```python
from build123d import *

# Parameters (mm, degrees)
F0_W     = 250
F0_H     = 100
F1_DEPTH = 5
F4_DEPTH = 50
F5_R     = 5
F6_R     = 4.99999


# Not quite as in the source:
# - two fillets or chamfers of one size are made in one step
# - a fillet or chamfer is up to 0.001 mm smaller than in the source, because OpenCascade refuses the exact size


with BuildPart() as f1:
    # F0 (on Front) → F1 (new body, symmetric)
    with BuildSketch(Plane.XZ):
        Rectangle(F0_W, F0_H)
    extrude(amount=F1_DEPTH, both=True)

    # F3 (on Top) → F4 (join, symmetric)
    with BuildSketch(Plane.XY):
        Polygon((-55.8243768029, -21.1299679096), (-77.5685643683, -5), (-94.3532884121, -5), (-61.7821750806, -29.1614459605), align=None)
    extrude(amount=F4_DEPTH, both=True)

    # F5
    f5_edges = [f1.edges().sort_by_distance(p)[0] for p in [
        (-94.353288, -5, 0),
        (-77.568564, -5, 0),
    ]]
    fillet(f5_edges, radius=F5_R)

    # F6 (radius 5 in the source; OpenCascade refuses exactly that, so slightly less here)
    f6_edges = [f1.edges().sort_by_distance(p)[0] for p in [
        (-61.782175, -29.161446, 0),
        (-55.824377, -21.129968, 0),
    ]]
    fillet(f6_edges, radius=F6_R)


solid = f1.part
```
Source: CAD feature listing. Evaluate the final solid. Frame: model axes, mm. A direction names the side the tool comes from. Round coordinates to 2 decimals unless told otherwise and drop trailing zeros. Loops run counter-clockwise (first coordinate to the right, second up) from the corner with the lowest first, then second, coordinate; pieces in that order, holes last. Notation, with made-up numbers: M -30,33.5 L -6,33.5 A28 ccw -6,56.5 Z; hole C -15.5,40 d6. An arc over 180 degrees is marked long. Use a Markdown table: item, result. Add a question column.
1. Section query B-B on x = -10. Return the cut outline in (y, z).
2. Line query: line 1 (Y direction, x = 87.5, z = -14); line 2 (Y direction, x = -63, z = 13); line 3 (X direction, y = -12.5, z = -29). Output: solid intervals per line, ascending.
3. Mould query, pull axis Y, two halves, no side actions, for faces 1 (the cylindrical face through (-62, -27.1, -0.7)), 2 (the cylindrical face through (-67.155, -8.348, 0.7)), 3 (the flat face through (-10, -2, 50)), 4 (the flat face through (-62.59, -16.11, 0.7)). Classes: pulls with the +Y half, pulls with the -Y half, needs draft (parallel to the pull), parting line crosses it, or undercut.
4. Contact query for flat-ended pins moving along their axis: P1, Ø10, axis at x = -66, z = -6, coming from the -Y side; P2, Ø14.5, axis at x = -104, z = -6.5, coming from the -Y side. Output: stop coordinate, or through.
5. Section query C-C on y = -21. Return the cut outline in (x, z), then the cut area to 3 significant figures.
6. Reachability of faces 5 (the cylindrical face through (-57.88, -21.38, -0.7)), 6 (the flat face through (-111, -5, 1)) from +Z, -Z, +X, -X, +Y, -Y: full face, straight path, thin tool, end or side. Return the list, or none.
Reported:
| question | item | result |
|---|---|---|
| 1 | outline | M -5,-50 L 5,-50 L 5,50 L -5,50 Z |
| 2 | line 1 | y = -5 to 5 |
| 2 | line 2 | y = -27.16 to -15.81, -5.03 to 5 |
| 2 | line 3 | x = -84.24 to -66.77 |
| 3 | face 1 | pulls with the -Y half |
| 3 | face 2 | undercut |
| 3 | face 3 | needs draft |
| 3 | face 4 | undercut |
| 4 | P1 | stops at y = -27.17 |
| 4 | P2 | stops at y = -5 |
| 5 | outline | M -72.78,-50 L -57.96,-50 L -57.96,50 L -72.78,50 Z |
| 5 | area | 1,480 mm² |
| 6 | face 5 | +Z, -Z, +X |
| 6 | face 6 | +Z, -Z, -X, -Y |
